Autodesk Inventor part; units mm, degrees
ref_plane "YZ Plane" through (0, 0, 0) normal (1, 0, 0) x (0, 1, 0)
ref_plane "XZ Plane" through (0, 0, 0) normal (0, 1, 0) x (-1, 0, 0)
ref_plane "XY Plane" through (0, 0, 0) normal (0, 0, 1) x (1, 0, 0)
sketch "Sketch10" plane through (0, 0, 0) normal (1, 0, 0) x (0, 1, 0)
  line L0 (0, 4) -> (1.7812, 4)
  line L1 (1.7812, 4) -> (6.4, -4)
  line L2 (6.4, -4) -> (0, -4)
  line L3 (0, -4) -> (0, 4)
  line L4 (0, 2.4) -> (1.32, 2.4)
  line L5 (1.32, 2.4) -> (4.0913, -2.4)
  line L6 (4.0913, -2.4) -> (0, -2.4)
  point P0 (0, 0)
  point P1 (0, 0)
  dimension "d91" = 8
  dimension "d92" = 6.4
  dimension "d103" = 30
  dimension "d109" = 1.32
  dimension "d110" = 1.6
  dimension "d111" = 1.6
extrude "Extrusion6" add sketch "Sketch10" along normal mid plane 8
sketch "Sketch11" plane through (-4, 0, -4) normal (0, -1, 0) x (1, 0, 0)
  line L0 (1.6, 6.4) -> (6.4, 6.4) construction
  line L1 (6.4, 6.4) -> (6.4, 1.6) construction
  line L2 (6.4, 1.6) -> (1.6, 1.6) construction
  line L3 (1.6, 1.6) -> (1.6, 6.4) construction
  circle A0 centre (4, 4) radius 2.4
  line L4 (8, 0) -> (0, 0)
  line L5 (8, 8) -> (8, 0)
  line L6 (0, 8) -> (8, 8)
  line L7 (0, 0) -> (0, 8)
  line L8 (0.4, 7.6) -> (7.6, 7.6)
  line L9 (7.6, 7.6) -> (7.6, 0.4)
  line L10 (7.6, 0.4) -> (0.4, 0.4)
  line L11 (0.4, 0.4) -> (0.4, 7.6)
  point P0 (0.4, 4)
  point P1 (4, 0.4)
  dimension "d96" = 4.8
  dimension "d104" = 0.4
  dimension "d105" = 0.4
extrude "Extrusion9" cut sketch "Sketch10" along normal mid plane 4.8 contours L4 L5 L6 L3
extrude "Extrusion7" cut sketch "Sketch11" against normal blind 1.6 contours A0
extrude "Extrusion8" cut sketch "Sketch11" against normal blind 0.4 contours L4 L7 L6 L5
fillet "Fillet1" radius 0.2 8 edges at (-4, 4.0906, 0) (0, 1.7812, 4) (-4, 1.0906, 4) (4, 1.0906, 4) (4, 4.0906, 0) (4, 3.4, -4) (0, 6.4, -4) (-4, 3.4, -4)
equation "\"d91\" = lu"
equation "\"d92\" = 0.666667 * lh"
equation "\"d110\" = wall"
equation "\"d111\" = d110"
equation "\"d94\" = lu"
equation "\"d96\" = kd"
equation "\"d104\" = gw"
equation "\"d105\" = gw"
equation "\"d112\" = lu - 2 * wall"
equation "\"d97\" = 0.333333 * lh - topthk"
equation "\"d106\" = gh"
equation "\"d22\" = 2 * lf"
properties part number "54200-TransClear" material "Polycarbonate"
The model under review builds one solid part; all positions refer to its coordinate system, in mm. A direction names the side the tool comes from. Round coordinates to 2 decimals unless told otherwise and drop trailing zeros. Order: outer loops, then holes, each group sorted by start corner. A loop starts at its lowest first (then second) coordinate and runs counter-clockwise, first axis right, second up. Notation, with made-up numbers: (-27, 53.25) - (23, 53.25) arc R19 cw to (23, 79.25) - close; hole circle Ø8 at (11, 87.5). An arc over 180 degrees is marked (long way). Answer in a Markdown table with one row per item.
(1) Clearance check with flat-ended pins moving along their axes: P1, Ø0.5, axis at x = 0, z = 2, coming from the -Y side; P2, Ø1.5, axis at x = 0.5, y = 5, coming from the +Z side. State where each tip first meets the part, or that it passes through.
Result set:
| item | result |
|---|---|
| P1 | stops at y = 1.6 |
| P2 | stops at z = -0.28 |
(2) Take a section at D-D on x = -1.25. Write out the cut boundary in (y, z).
Result set:
| item | result |
|---|---|
| outline | (0, -3.6) - (0.4, -3.6) - (0.4, -4) - (6.05, -4) arc R0.2 ccw to (6.23, -3.7) - (1.84, 3.9) arc R0.2 ccw to (1.67, 4) - (0.4, 4) - (0.4, 3.6) - (0, 3.6) - (0, 2.4) - (1.32, 2.4) - (1.52, 2.05) - (1.6, 2.05) - (1.6, 1.92) - (4.09, -2.4) - (0, -2.4) - close |
(3) Take a section at C-C on x = 1.75. Write out the cut boundary in (y, z).
Result set:
| item | result |
|---|---|
| outline | (0, -3.6) - (0.4, -3.6) - (0.4, -4) - (6.05, -4) arc R0.2 ccw to (6.23, -3.7) - (1.84, 3.9) arc R0.2 ccw to (1.67, 4) - (0.4, 4) - (0.4, 3.6) - (0, 3.6) - (0, 2.4) - (1.32, 2.4) - (4.09, -2.4) - (0, -2.4) - close |
(4) Machinability: for faces 1 (the face through (-0.053, 4.002, 0.153)), 2 (the face through (0, 1, 2.4)), which of the approach directions +Z, -Z, +X, -X, +Y, -Y give a long, thin tool a straight path to every point of the face, cutting with its end or side? Answer none if there is none.
Result set:
| item | result |
|---|---|
| face 1 | +Z, +X, -X, +Y |
| face 2 | -Y |
(5) For line 1 (X direction, y = 1.25, z = -0.5); line 2 (Z direction, x = -2, y = 1.5); line 3 (Z direction, x = -2.25, y = 2), list the stretches that pass through material, from the lowest coordinate up. Write a range as from..to.
Result set:
| item | result |
|---|---|
| line 1 | x = -4..-2.4, 2.4..4 |
| line 2 | z = -4..-2.4, 2.09..4 |
| line 3 | z = -4..-2.4, 1.22..3.62 |
(6) Mouldability with a two-part tool opening along X and no side actions: class faces 3 (the face through (2.4, 2, 0)), 4 (the face through (0, 3, -4)), 5 (the face through (3.94, 4.01, 0.02)) as released by +X, released by -X, zero draft, split by the parting line, or undercut.
Result set:
| item | result |
|---|---|
| face 3 | undercut |
| face 4 | zero draft |
| face 5 | released by +X |
(7) Take a section at B-B on x = -3. Write out the cut boundary in (y, z), plus the area to 3 significant figures.
Result set:
| item | result |
|---|---|
| outline | (0, -3.6) - (0.4, -3.6) - (0.4, -4) - (6.05, -4) arc R0.2 ccw to (6.23, -3.7) - (1.84, 3.9) arc R0.2 ccw to (1.67, 4) - (0.4, 4) - (0.4, 3.6) - (0, 3.6) - close |
| area | 32.4 mm2 |
(8) Take a section at A-A on y = 1. Write out the cut boundary in (x, z).
Result set:
| item | result |
|---|---|
| outline | (-4, -3.8) arc R0.2 ccw to (-3.8, -4) - (3.8, -4) arc R0.2 ccw to (4, -3.8) - (4, 3.8) arc R0.2 ccw to (3.8, 4) - (-3.8, 4) arc R0.2 ccw to (-4, 3.8) - close; hole (-2.4, -2.4) - (2.4, -2.4) - (2.4, 2.4) - (-2.4, 2.4) - close |
